```python
from build123d import *

# Parameters (mm, degrees)
SKETCH1_W               = 70
SKETCH1_H               = 50
BOSS_EXTRUDE1_DEPTH     = 6
SHELL1_T                = -3
FILLET1_R               = 5
FILLET2_R               = 5
FILLET3_R               = 5
FILLET4_R               = 5
FILLET5_R               = 5
FILLET6_R               = 5
FILLET7_R               = 5
FILLET8_R               = 5
FILLET9_R               = 5
SKETCH2_W               = 12
SKETCH2_H               = 40
CUT_EXTRUDE1_DEPTH      = 10
CUT_EXTRUDE1_DEPTH_BACK = 10


with BuildPart() as part:
    # Sketch1 → Boss-Extrude1 (new body)
    with BuildSketch(Plane(origin=(0, 0, 0), x_dir=(1, 0, 0), z_dir=(0, 1, 0))):
        Rectangle(SKETCH1_W, SKETCH1_H)
    extrude(amount=BOSS_EXTRUDE1_DEPTH)

    # Shell1
    shell1_openings = [part.faces().sort_by_distance(p)[0] for p in [
        (0, 6, 0),
    ]]
    offset(amount=SHELL1_T, openings=shell1_openings, kind=Kind.INTERSECTION)

    # Fillet1
    fillet1_edges = [part.edges().sort_by_distance(p)[0] for p in [
        (35, 3, 25),
    ]]
    fillet(fillet1_edges, radius=FILLET1_R)

    # Fillet2
    fillet2_edges = [part.edges().sort_by_distance(p)[0] for p in [
        (35, 3, -25),
    ]]
    fillet(fillet2_edges, radius=FILLET2_R)

    # Fillet3
    fillet3_edges = [part.edges().sort_by_distance(p)[0] for p in [
        (-35, 3, 25),
    ]]
    fillet(fillet3_edges, radius=FILLET3_R)

    # Fillet4
    fillet4_edges = [part.edges().sort_by_distance(p)[0] for p in [
        (-35, 3, -25),
    ]]
    fillet(fillet4_edges, radius=FILLET4_R)

    # Fillet5
    fillet5_edges = [part.edges().sort_by_distance(p)[0] for p in [
        (35, 0, 0),
        (0, 0, -25),
        (0, 0, 25),
        (-35, 0, 0),
    ]]
    fillet(fillet5_edges, radius=FILLET5_R)

    # Fillet6
    fillet6_edges = [part.edges().sort_by_distance(p)[0] for p in [
        (32, 4.5, 22),
    ]]
    fillet(fillet6_edges, radius=FILLET6_R)

    # Fillet7
    fillet7_edges = [part.edges().sort_by_distance(p)[0] for p in [
        (-32, 4.5, 22),
    ]]
    fillet(fillet7_edges, radius=FILLET7_R)

    # Fillet8
    fillet8_edges = [part.edges().sort_by_distance(p)[0] for p in [
        (-32, 4.5, -22),
    ]]
    fillet(fillet8_edges, radius=FILLET8_R)

    # Fillet9
    fillet9_edges = [part.edges().sort_by_distance(p)[0] for p in [
        (32, 4.5, -22),
    ]]
    fillet(fillet9_edges, radius=FILLET9_R)

    # Sketch2 → Cut-Extrude1 (cut, two sides)
    with BuildSketch(Plane.XZ) as cut_extrude1_sk:
        with Locations((-24, 0)):
            Rectangle(SKETCH2_W, SKETCH2_H)
    extrude(amount=CUT_EXTRUDE1_DEPTH, mode=Mode.SUBTRACT)
    extrude(cut_extrude1_sk.sketch, amount=-CUT_EXTRUDE1_DEPTH_BACK, mode=Mode.SUBTRACT)


solid = part.part
```
Design review of the part built by this model. Coordinates are the model's own, in mm. A direction names the side the tool comes from. Coordinates: 2 decimals unless noted, no trailing zeros. Loops run counter-clockwise (first coordinate to the right, second up) from the corner with the lowest first, then second, coordinate; pieces in that order, holes last.
Q1. We need section A-A on z = 3.5. State the section outline as (x, y) points.
Reported:
outline: (-35, 5) arc R5 ccw to (-30, 0) - (-30, 3) - (-32, 3) - (-32, 6) - (-35, 6) - close; (-18, 0) - (30, 0) arc R5 ccw to (35, 5) - (35, 6) - (32, 6) - (32, 3) - (-18, 3) - close
Q2. Tool access review of faces 1 (the face through (-24, 1, -20)), 2 (the face through (33.57, 5.51, -23.5)), 3 (the face through (0, 4, 22)): name each direction out of +Z, -Z, +X, -X, +Y, -Y from which nothing blocks a thin tool from reaching the whole face with its end or side.
Reported:
face 1: +Y, -Y
face 2: -Z, +X, +Y, -Y
face 3: +Y
Q3. For pin 1 (6 mm diameter, centred on x = 0.5, z = 9, fed in from +Y); pin 2 (1.5 mm diameter, centred on y = 2, z = 2.5, fed in from +X); pin 3 (0.9 mm diameter, centred on y = 4, z = 7.5, fed in from -X), all flat-tipped, find the tip position at first contact; note any pin that passes through.
Reported:
pin 1: stops at y = 3
pin 2: stops at x = 34.47
pin 3: stops at x = -34.97
Q4. We need section B-B on y = 2. State the section outline as (x, z) points, and give its area (3 significant figures).
Reported:
outline: (-34, -20) arc R4 ccw to (-30, -24) - (30, -24) arc R4 ccw to (34, -20) - (34, 20) arc R4 ccw to (30, 24) - (-30, 24) arc R4 ccw to (-34, 20) - close; hole (-30, -20) - (-18, -20) - (-18, 20) - (-30, 20) - close
area: 2,770 mm2
Q5. To check wall thickness, follow line 1 (X direction, y = 4.75, z = -1); line 2 (Y direction, x = 17, z = 7.5); line 3 (Z direction, x = 7.5, y = 4.25). State the ranges of each line that lie inside material, in increasing order.
Reported:
line 1: x = -34.99 to -32, 32 to 34.99
line 2: y = 0 to 3
line 3: z = -24.94 to -22, 22 to 24.94
Q6. The part is to be moulded in two halves that separate along X. For faces 4 (the face through (-33.57, 5.51, -23.5)), 5 (the face through (33.5, 5.51, 23.57)), 6 (the face through (0, 1, 23)), 7 (the face through (32, 4, 0)), say which applies: +X half, -X half, draft (parallel to the pull), parting line (faces both ways), or undercut.
Reported:
face 4: -X half
face 5: +X half
face 6: draft
face 7: undercut
Q7. We need section C-C on x = -23. State the section outline as (y, z) points, and give its area (3 significant figures).
Reported:
outline: (0, -20) arc R5 ccw to (5, -25) - (6, -25) - (6, -22) - (3, -22) - (3, -20) - close; (0, 20) - (3, 20) - (3, 22) - (6, 22) - (6, 25) - (5, 25) arc R5 ccw to start
area: 37.3 mm2
Q8. We need section D-D on x = -15. State the section outline as (y, z) points.
Reported:
outline: (0, -20) arc R5 ccw to (5, -25) - (6, -25) - (6, -22) - (3, -22) - (3, 22) - (6, 22) - (6, 25) - (5, 25) arc R5 ccw to (0, 20) - close
